```python
from build123d import *

# Parameters (mm, degrees)
SKETCH1_W                  = 15.9
SKETCH1_H                  = 15.8
BOSS_EXTRUDE1_DEPTH        = 3.2
BOSS_EXTRUDE1_TAPER        = 1
SKETCH2_R                  = 2.4
BOSS_EXTRUDE2_DEPTH        = 1.8
CHAMFER3_SIZE              = 0.25
LPATTERN2_COUNT            = 2
LPATTERN2_PITCH            = 8
LPATTERN2_COUNT_DIR2       = 2
LPATTERN2_PITCH_DIR2       = 8
CHAMFER3_OF_LPATTERN2_SIZE = 0.25
SHELL1_OUTLINE_R           = 1.2
SHELL1_DEPTH               = 3.8
FILLET2_R                  = 0.25


with BuildPart() as part:
    # Sketch1 → Boss-Extrude1 (new body)
    with BuildSketch(Plane.XY):
        Rectangle(SKETCH1_W, SKETCH1_H)
    extrude(amount=BOSS_EXTRUDE1_DEPTH, taper=BOSS_EXTRUDE1_TAPER)

    # Sketch2 → Boss-Extrude2 (add)
    with BuildSketch(Plane.XY.offset(3.2)):
        with Locations(Location((-4.05, -4, 0), (0, 0, 180))):
            Circle(SKETCH2_R)
    boss_extrude2 = extrude(amount=BOSS_EXTRUDE2_DEPTH)

    # Chamfer3
    chamfer3_edges = [part.edges().sort_by_distance(p)[0] for p in [
        (-1.65, -4, 5),
    ]]
    chamfer(chamfer3_edges, length=CHAMFER3_SIZE)

    # LPattern2: Boss-Extrude2 2 × 2
    with Locations(*[(j * LPATTERN2_PITCH_DIR2, i * LPATTERN2_PITCH, 0) for i in range(LPATTERN2_COUNT) for j in range(LPATTERN2_COUNT_DIR2) if (i, j) != (0, 0)]):
        add(boss_extrude2)

    # Chamfer3 of LPattern2
    chamfer3_of_lpattern2_edges = [part.edges().sort_by_distance(p)[0] for p in [
        (6.35, -4, 5),
        (-1.65, 4, 5),
        (6.35, 4, 5),
    ]]
    chamfer(chamfer3_of_lpattern2_edges, length=CHAMFER3_OF_LPATTERN2_SIZE)

    # Shell1: read off the stored shape, not the designer's step
    # Shell1 outline → Shell1 (cut)
    with BuildSketch(Plane.XY):
        with Locations((3.95, 4)):
            Circle(SHELL1_OUTLINE_R)
        with Locations((3.95, -4)):
            Circle(SHELL1_OUTLINE_R)
        with Locations((-4.05, -4)):
            Circle(SHELL1_OUTLINE_R)
        with Locations((-4.05, 4)):
            Circle(SHELL1_OUTLINE_R)
    extrude(amount=SHELL1_DEPTH, mode=Mode.SUBTRACT)

    # Shell1 2: loft between two sections, ruled curve by curve
    shell1_2_from = [
        Edge.make_line((-6.714907076, 6.664907076, 2), (-6.714907076, -6.664907076, 2)),
        Edge.make_line((-6.714907076, -6.664907076, 2), (6.714907076, -6.664907076, 2)),
        Edge.make_line((6.714907076, -6.664907076, 2), (6.714907076, 6.664907076, 2)),
        Edge.make_line((6.714907076, 6.664907076, 2), (-6.714907076, 6.664907076, 2)),
    ]
    shell1_2_to = [
        Edge.make_line((-6.749817206, 6.699817206, 0), (-6.749817206, -6.699817206, 0)),
        Edge.make_line((-6.749817206, -6.699817206, 0), (6.749817206, -6.699817206, 0)),
        Edge.make_line((6.749817206, -6.699817206, 0), (6.749817206, 6.699817206, 0)),
        Edge.make_line((6.749817206, 6.699817206, 0), (-6.749817206, 6.699817206, 0)),
    ]
    shell1_2 = Solid(Shell([*[Face.make_surface_from_curves(shell1_2_from[k], shell1_2_to[k]) for k in range(4)], Face(Wire(shell1_2_from)), Face(Wire(shell1_2_to))]))
    add(shell1_2, mode=Mode.SUBTRACT)

    # Fillet2
    fillet2_edges = [part.edges().sort_by_distance(p)[0] for p in [
        (7.894143792, 0, 3.2),
        (0, 7.844143792, 3.2),
        (-1.65, -4, 3.2),
        (-1.65, 4, 3.2),
        (6.35, -4, 3.2),
        (6.35, 4, 3.2),
        (-7.894143792, 0, 3.2),
        (-7.922071434, 7.872071434, 1.600026465),
        (7.922071896, 7.872071896, 1.6),
        (7.922071434, -7.872071434, 1.600026465),
        (-7.922071896, -7.872071896, 1.6),
        (0, -7.844143792, 3.2),
    ]]
    fillet(fillet2_edges, radius=FILLET2_R)


solid = part.part
```
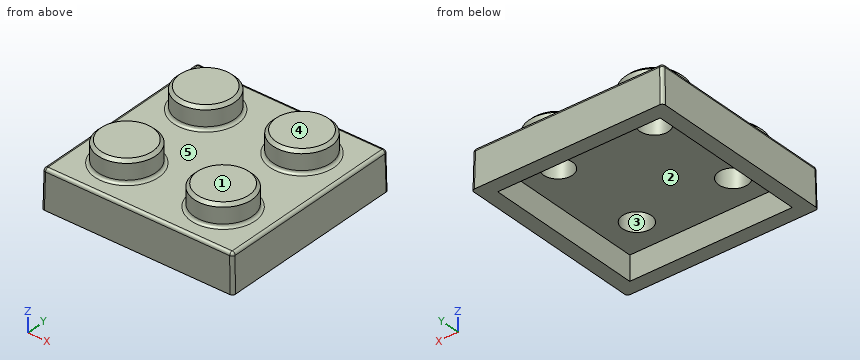
The model under review builds one solid part; all positions refer to its coordinate system, in mm. Face numbers are marked on the shaded views. A direction names the side the tool comes from. Coordinates: 2 decimals unless noted, no trailing zeros. Order: outer loops, then holes, each group sorted by start corner. A loop starts at its lowest first (then second) coordinate and runs counter-clockwise, first axis right, second up. Notation, with made-up numbers: (54, 55) -> (67, 55) arc R4 cw to (67, 61) -> close; hole circle Ø3 at (-9, 33). An arc over 180 degrees is marked (long way). Answer in a Markdown table with one row per item. Add a question column.
Item 1: We need section A-A on x = -7. Write out the cut boundary in (y, z), plus the area to 3 significant figures.
Item 2: Clearance check with flat-ended pins moving along their axes: pin 1 (1.2 mm diameter, centred on x = 4.5, y = 4, fed in from -Z); pin 2 (2 mm diameter, centred on x = -4, z = 1.5, fed in from -Y); pin 3 (2 mm diameter, centred on y = -5, z = 1.5, fed in from -X). State where each tip first meets the part, or that it passes through.
Item 3: We need section B-B on z = 2.2. Give the number of separate pieces and of enclosed holes in the cut face, plus the area to 3 significant figures.
Item 4: Mouldability with a two-part tool opening along X and no side actions: class the marked faces 1 and 2 as +X half, -X half, draft (parallel to the pull), parting line (faces both ways), or undercut.
Item 5: Machinability: for the marked faces 3, 4 and 5, which of the approach directions +Z, -Z, +X, -X, +Y, -Y give a long, thin tool a straight path to every point of the face, cutting with its end or side? Answer none if there is none.
Item 6: To check wall thickness, follow probe 1 along Y at (x, z) = (3.95, 2.95); probe 2 along X at (y, z) = (4.5, 2.45). State the ranges of each line that lie inside material, in increasing order.
Final values:
| question | item | result |
|---|---|---|
| 1 | outline | (-7.9, 0) -> (7.9, 0) -> (7.85, 2.95) arc R0.25 ccw to (7.6, 3.2) -> (-7.6, 3.2) arc R0.25 ccw to (-7.85, 2.95) -> close |
| 1 | area | 50.4 mm2 |
| 2 | pin 1 | stops at z = 3.8 |
| 2 | pin 2 | stops at y = -7.89 |
| 2 | pin 3 | stops at x = -7.94 |
| 3 | separate pieces | 1 |
| 3 | enclosed holes | 4 |
| 3 | area | 231 mm2 |
| 4 | face 1 | draft |
| 4 | face 2 | undercut |
| 5 | face 3 | -Z |
| 5 | face 4 | +Z, +X, -X, +Y, -Y |
| 5 | face 5 | +Z |
| 6 | probe 1 | y = -7.85 to -5.2, -2.8 to 2.8, 5.2 to 7.85 |
| 6 | probe 2 | x = -7.91 to -5.14, -2.96 to 2.86, 5.04 to 7.91 |
